Can you work these out from the model? Positions are in its coordinate system, mm. Coordinates: 2 decimals unless noted, no trailing zeros. Order: outer loops, then holes, each group sorted by start corner. A loop starts at its lowest first (then second) coordinate and runs counter-clockwise, first axis right, second up. Notation, with made-up numbers: (-34, 32) -> (-6, 32) arc R21 cw to (-6, 53) -> close; hole circle Ø8 at (-33, 74.25). An arc over 180 degrees is marked (long way). Answer in a Markdown table with one row per item.
```python
from build123d import *

# Parameters (mm, degrees)
F1_DEPTH = 76.2
F3_SIZE  = 5.08


# Not quite as in the source:
# - the program builds the solid bodies; features that only make, move or delete a surface that nothing else refers to are left out


with BuildPart() as f1:
    # F0 (on Top) → F1 (new body)
    with BuildSketch(Plane.XY):
        with BuildLine():
            ThreePointArc((0, 37.8345108272), (26.7530391688, 26.7530391688), (37.8345108272, 0))
            Line((37.8345108272, 0), (129.7342181206, 0))
            Line((129.7342181206, 0), (129.7342181206, 58.8485188782))
            Line((129.7342181206, 58.8485188782), (0, 58.8485188782))
            Line((0, 58.8485188782), (0, 37.8345108272))
        make_face()
    extrude(amount=F1_DEPTH)

    # F3
    f3_edges = [f1.edges().sort_by_distance(p)[0] for p in [
        (129.734218, 29.424259, 0),
    ]]
    chamfer(f3_edges, length=F3_SIZE)


solid = f1.part
```
(1) Suppose I cut it at A-A (y = 27). Please give me the cut outline in (x, z).
Response values:
| item | result |
|---|---|
| outline | (26.5, 0) -> (124.65, 0) -> (129.73, 5.08) -> (129.73, 76.2) -> (26.5, 76.2) -> close |
(2) I need wall thicknesses on line 1 (X direction, y = 5.5, z = 60); line 2 (X direction, y = 8, z = 31); line 3 (Y direction, x = 14, z = 45.5). Which ranges of each line are inside material? Lowest first, please. Write a range as [from, to].
Response values:
| item | result |
|---|---|
| line 1 | [37.43, 129.73] |
| line 2 | [36.98, 129.73] |
| line 3 | [35.15, 58.85] |
(3) Suppose I cut it at C-C (x = 8.5). Please give me the cut outline in (y, z), and give its area (3 significant figures).
Response values:
| item | result |
|---|---|
| outline | (36.87, 0) -> (58.85, 0) -> (58.85, 76.2) -> (36.87, 76.2) -> close |
| area | 1,670 mm2 |
(4) Suppose I cut it at B-B (z = 69). Please give me the cut outline in (x, y).
Response values:
| item | result |
|---|---|
| outline | (0, 37.83) arc R37.83 cw to (37.83, 0) -> (129.73, 0) -> (129.73, 58.85) -> (0, 58.85) -> close |
